from build123d import *

# Parameters (mm, degrees)
F0_W      = 152.4
F0_H      = 152.4
F1_DEPTH  = 19.05
F2_R      = 4.3815
F3_DEPTH  = 19.05
F4_R      = 4.6355
F5_DEPTH  = 0.508
F6_R      = 1.1303
F8_DEPTH  = 6.35
F9_DEPTH  = 9.525
F10_R     = 1.1303
F11_DEPTH = 19.05
F12_R     = 4.7625
F13_DEPTH = 3.175
F14_R     = 1.1303
F15_DEPTH = 9.525


with BuildPart() as f1:
    # F0 (on Top) → F1 (new body)
    with BuildSketch(Plane.XY):
        Rectangle(F0_W, F0_H)
    extrude(amount=F1_DEPTH)

    # F2 (on face) → F3 (cut, through all)
    with BuildSketch(Plane.XY.offset(19.05)):
        with Locations((-66.675, 66.675)):
            Circle(F2_R)
        with Locations((-66.675, -66.675)):
            Circle(F2_R)
        with Locations((66.675, -66.675)):
            Circle(F2_R)
    extrude(amount=-F3_DEPTH, mode=Mode.SUBTRACT)

    # F4 (on face) → F5 (cut)
    with BuildSketch(Plane.XY.offset(19.05)):
        with Locations((-66.675, 66.675)):
            Circle(F4_R)
        with Locations((-66.675, -66.675)):
            Circle(F4_R)
        with Locations((66.675, -66.675)):
            Circle(F4_R)
    extrude(amount=-F5_DEPTH, mode=Mode.SUBTRACT)

    # F6 (on face) → F8 (cut)
    with BuildSketch(Plane.XY.offset(19.05)):
        with Locations((-31.75, 31.75)):
            Circle(F6_R)
        with Locations((31.75, 31.75)):
            Circle(F6_R)
        with Locations((31.75, -31.75)):
            Circle(F6_R)
        with Locations((-31.75, -31.75)):
            Circle(F6_R)
    extrude(amount=-F8_DEPTH, mode=Mode.SUBTRACT)

    # F7 (on face) → F9 (cut)
    with BuildSketch(Plane.XY.offset(19.05)):
        with BuildLine():
            ThreePointArc((20.828, -35.306), (14.351, -28.829), (20.828, -22.352))
            Line((20.828, -22.352), (-20.828, -22.352))
            ThreePointArc((-20.828, -22.352), (-16.2480693783, -24.2490693783), (-14.351, -28.829))
            ThreePointArc((-14.351, -28.829), (-16.2480693783, -33.4089306217), (-20.828, -35.306))
            Line((-20.828, -35.306), (20.828, -35.306))
        make_face()
        with BuildLine():
            ThreePointArc((27.305, -28.829), (25.4079306217, -24.2490693783), (20.828, -22.352))
            Line((20.828, -22.352), (20.828, -35.306))
            ThreePointArc((20.828, -35.306), (25.4079306217, -33.4089306217), (27.305, -28.829))
        make_face()
        with BuildLine():
            Line((20.828, -35.306), (20.828, -22.352))
            ThreePointArc((20.828, -22.352), (14.351, -28.829), (20.828, -35.306))
        make_face()
        with BuildLine():
            ThreePointArc((-14.351, -28.829), (-16.2480693783, -24.2490693783), (-20.828, -22.352))
            Line((-20.828, -22.352), (-20.828, -35.306))
            ThreePointArc((-20.828, -35.306), (-16.2480693783, -33.4089306217), (-14.351, -28.829))
        make_face()
        with BuildLine():
            Line((-20.828, -35.306), (-20.828, -22.352))
            ThreePointArc((-20.828, -22.352), (-27.305, -28.829), (-20.828, -35.306))
        make_face()
        with BuildLine():
            ThreePointArc((-6.477, -12.7), (0, -19.177), (6.477, -12.7))
            Line((6.477, -12.7), (-6.477, -12.7))
        make_face()
        with BuildLine():
            ThreePointArc((-6.477, -12.7), (0, -6.223), (6.477, -12.7))
            Line((6.477, -12.7), (6.477, 28.956))
            ThreePointArc((6.477, 28.956), (0, 22.479), (-6.477, 28.956))
            Line((-6.477, 28.956), (-6.477, -12.7))
        make_face()
        with BuildLine():
            Line((-6.477, -12.7), (6.477, -12.7))
            ThreePointArc((6.477, -12.7), (0, -6.223), (-6.477, -12.7))
        make_face()
        with BuildLine():
            ThreePointArc((-6.477, 28.956), (0, 22.479), (6.477, 28.956))
            Line((6.477, 28.956), (-6.477, 28.956))
        make_face()
        with BuildLine():
            Line((-6.477, 28.956), (6.477, 28.956))
            ThreePointArc((6.477, 28.956), (0, 35.433), (-6.477, 28.956))
        make_face()
    extrude(amount=-F9_DEPTH, mode=Mode.SUBTRACT)

    # F10 (on face) → F11 (cut, through all)
    with BuildSketch(Plane.XY.offset(19.05)):
        with Locations((0, -4.572)):
            Circle(F10_R)
        with Locations((0, 20.828)):
            Circle(F10_R)
        with Locations((-12.7, -28.829)):
            Circle(F10_R)
        with Locations((12.7, -28.829)):
            Circle(F10_R)
    extrude(amount=-F11_DEPTH, mode=Mode.SUBTRACT)

    # F12 (on face) → F13 (cut)
    with BuildSketch(Plane(origin=(0, 0, 0), x_dir=(1, 0, 0), z_dir=(0, 0, -1))):
        with Locations((-12.7, 28.829)):
            Circle(F12_R)
        with Locations((12.7, 28.829)):
            Circle(F12_R)
        with Locations((0, 4.572)):
            Circle(F12_R)
        with Locations((0, -20.828)):
            Circle(F12_R)
    extrude(amount=-F13_DEPTH, mode=Mode.SUBTRACT)

    # F14 (on face) → F15 (cut)
    with BuildSketch(Plane.XY.offset(19.05)):
        with Locations((0, -66.675)):
            Circle(F14_R)
        with Locations((36.0472265039, -56.0905793015)):
            Circle(F14_R)
        with Locations((60.6497132903, -27.6977959919)):
            Circle(F14_R)
        with Locations((65.9963446374, 9.4888418419)):
            Circle(F14_R)
        with Locations((50.3896028701, 43.6628394358)):
            Circle(F14_R)
        with Locations((18.7845182274, 63.9741940157)):
            Circle(F14_R)
        with Locations((-18.7845182274, 63.9741940157)):
            Circle(F14_R)
        with Locations((-50.3896028701, 43.6628394358)):
            Circle(F14_R)
        with Locations((-65.9963446374, 9.4888418419)):
            Circle(F14_R)
        with Locations((-60.6497132903, -27.6977959919)):
            Circle(F14_R)
        with Locations((-36.0472265039, -56.0905793015)):
            Circle(F14_R)
    extrude(amount=-F15_DEPTH, mode=Mode.SUBTRACT)

    # F17 (on Front) → F18 (revolve, cut)
    with BuildSketch(Plane.XZ):
        Polygon((-53.1876, 19.05), (-60.6104428426, 19.05), (-60.3788214213, 14.6304), (-53.4192214213, 14.6304), align=None)
    revolve(axis=Axis((0, 0, 42.1973057091), (0, 0, 1)), mode=Mode.SUBTRACT)


solid = f1.part
Can you work these out from the model? Positions are in its coordinate system, mm. A direction names the side the tool comes from. Give positions to 0.01 mm unless a question says otherwise; leave off trailing zeros. One line per item, written item: value.
(1) I need wall thicknesses on line 1 along Y through (x, z) = (0, 0.7); line 2 along X through (y, z) = (-4.5, 12.5); line 3 along Y through (x, z) = (-31.75, 15). Which ranges of each line are inside material? Lowest first, please.
Verdict:
line 1: -76.2 to -9.33, 0.19 to 16.07, 25.59 to 76.2
line 2: -76.2 to -6.48, 6.48 to 76.2
line 3: -76.2 to -51.38, -42.94 to -32.88, -30.62 to 30.62, 32.88 to 42.94, 51.38 to 76.2
(2) On a 3-axis mill with a long thin cutter (end or side, diameter ignored), from which of +Z, -Z, +X, -X, +Y, -Y can I reach the whole of each face in a straight line? I mean faces 1 (the face through (-1, 1, 0)), 2 (the face through (14, -28, 3.175)), 3 (the face through (0.14, 35.43, 14.35)). Say none if no direction works.
Verdict:
face 1: -Z, +X, -X, +Y, -Y
face 2: -Z
face 3: +Z
(3) I'm going to push flat-ended pins straight in: pin 1 (6 mm diameter, centred on x = -57, y = 29, fed in from -Z); pin 2 (6 mm diameter, centred on x = 52.5, y = -22.5, fed in from +Z); pin 3 (2 mm diameter, centred on x = 0, y = 20.828, fed in from -Z); pin 4 (12.5 mm diameter, centred on x = 12.7, y = -28.829, fed in from +Z) (3 decimals). Where does each tip first touch, or does it pass through?
Verdict:
pin 1: z = 0
pin 2: z = 14.63
pin 3: through
pin 4: z = 9.525
(4) If we mould it in two halves opening along Y, with no side actions, what happens to faces 4 (the face through (-76.2, -1, 9)), 5 (the face through (-64.54, -70.79, 18.8)), 6 (the face through (-1, 76.2, 9))? For each: released by +Y, released by -Y, zero draft, split by the parting line, or undercut.
Verdict:
face 4: zero draft
face 5: undercut
face 6: released by +Y
(5) If we section it at A-A, the plane z = 16.5: State how many separate pieces and enclosed holes the cut face has, plus the area to 3 significant figures.
Verdict:
separate pieces: 2
enclosed holes: 21
area: 19,100 mm^2
